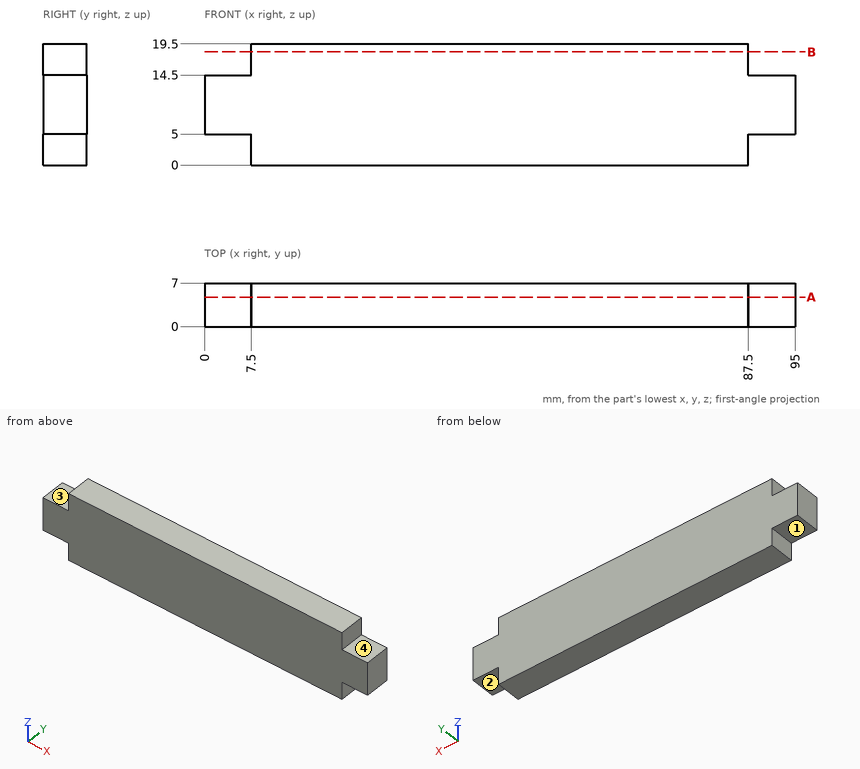
Verification items for this drawing (mm, ordinates from the low corner). A direction names the side the tool comes from. Give positions to 0.01 mm unless a question says otherwise; leave off trailing zeros. Loops run counter-clockwise (first coordinate to the right, second up) from the corner with the lowest first, then second, coordinate; pieces in that order, holes last.
(1) Set-up check for the marked faces 1, 2, 3 and 4: record each of +Z, -Z, +X, -X, +Y, -Y from which the full face is reachable in a straight line by a thin tool's end or side.
From the geometry:
face 1: -Z, -X, +Y, -Y
face 2: -Z, +X, +Y, -Y
face 3: +Z, -X, +Y, -Y
face 4: +Z, +X, +Y, -Y
(2) Section check A-A on y = 4.75. Record the cut outline in (x, z), then the cut area to 3 significant figures.
From the geometry:
outline: (0, 5) - (7.5, 5) - (7.5, 0) - (87.5, 0) - (87.5, 5) - (95, 5) - (95, 14.5) - (87.5, 14.5) - (87.5, 19.5) - (7.5, 19.5) - (7.5, 14.5) - (0, 14.5) - close
area: 1,700 mm2
(3) Section check B-B on z = 18.25. Record the cut outline in (x, y), then the cut area to 3 significant figures.
From the geometry:
outline: (7.5, 0) - (87.5, 0) - (87.5, 7) - (7.5, 7) - close
area: 560 mm2
(4) Depth check by flat-ended pin: pin 1 Ø2.5 at (y, z) = (3.5, 17.5) entering from -X; pin 2 Ø1.5 at (y, z) = (3.5, 18) entering from +X; pin 3 Ø3.5 at (x, y) = (3, 3.5) entering from +Z. Enter the tip coordinate at first touch or a pass-through.
From the geometry:
pin 1: stops at x = 7.5
pin 2: stops at x = 87.5
pin 3: stops at z = 14.5
(5) Thickness scan on L1, parallel to X at y = 1.75, z = 14.75. Record the ranges inside material, lowest first.
From the geometry:
L1: x = 7.5 to 87.5
